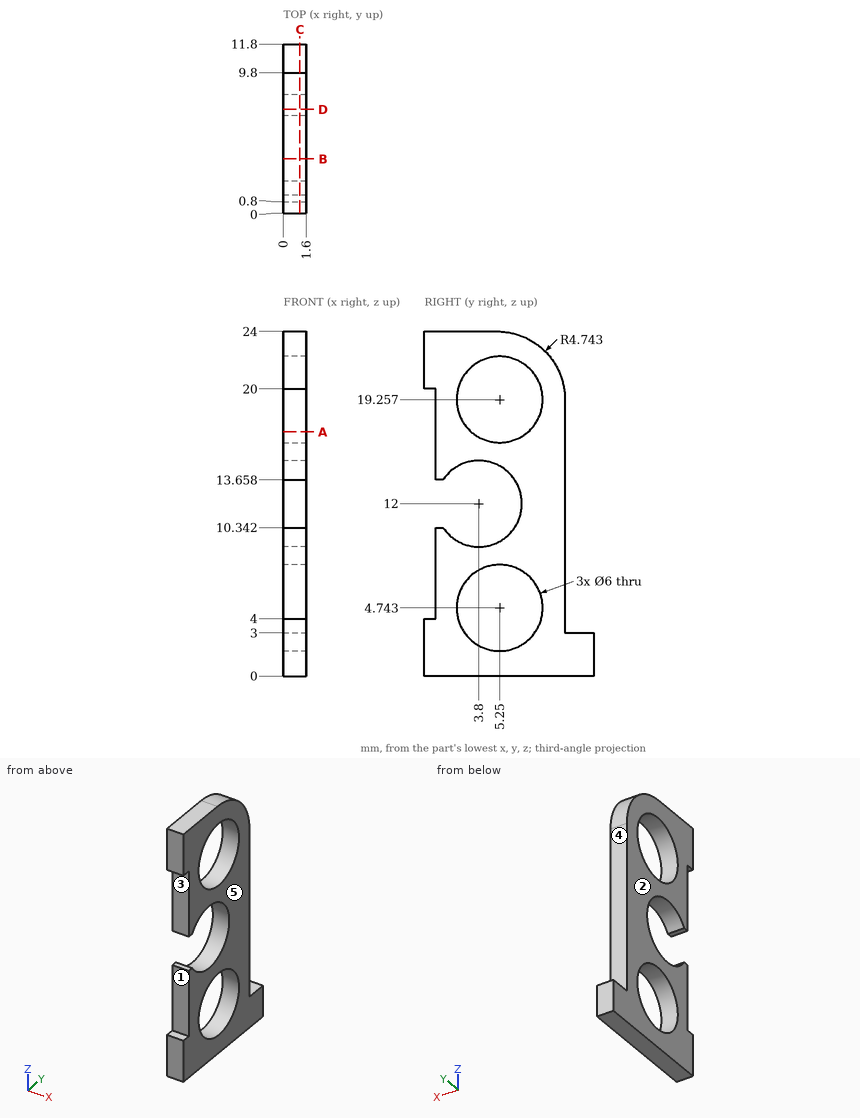
For this review, use the dimensioned drawing (mm, ordinates from the lowest corner) and the shaded views. A direction names the side the tool comes from. Round coordinates to 2 decimals unless told otherwise and drop trailing zeros. Order: outer loops, then holes, each group sorted by start corner. A loop starts at its lowest first (then second) coordinate and runs counter-clockwise, first axis right, second up. Notation, with made-up numbers: M -8.5,75 L 45.5,75 A30 ccw 45.5,110 Z; hole C 64,19.5 d6. An arc over 180 degrees is marked long. Use a Markdown table: item, result. Add a question column.
Item 1: Tool access review of the marked faces 3, 4 and 5: name each direction out of +Z, -Z, +X, -X, +Y, -Y from which nothing blocks a thin tool from reaching the whole face with its end or side.
Item 2: Add section A-A, the plane z = 17. Give the boundary of the cut face in (x, y).
Item 3: To check wall thickness, follow line 1 along Z through (x, y) = (0.55, 1.25); line 2 along Z through (x, y) = (0.55, 4.25) (1 decimal); line 3 along Z through (x, y) = (0.85, 11.25). State the ranges of each line that lie inside material, in increasing order.
Item 4: Add section B-B, the plane y = 3.8. Give the boundary of the cut face in (x, z), then the cut area to 3 significant figures.
Item 5: Add section C-C, the plane x = 1.15. Give the boundary of the cut face in (y, z), then the cut area to 3 significant figures.
Item 6: Insertion check: pin 1 (5 mm diameter, centred on y = 3.8, z = 12, fed in from -X). The pin has a flat end and moves straight along its axis. Give the tip position at first contact, or say it passes through.
Item 7: Add section D-D, the plane y = 7.25. Give the boundary of the cut face in (x, z).
Item 8: Mouldability with a two-part tool opening along Z and no side actions: class the marked faces 1 and 2 as released by +Z, released by -Z, zero draft, split by the parting line, or undercut.
Geometry results:
| question | item | result |
|---|---|---|
| 1 | face 3 | +X, -X, -Y |
| 1 | face 4 | +Z, +X, -X, +Y |
| 1 | face 5 | +Z, -Z, +X, +Y, -Y |
| 2 | outline | M 0,0.8 L 1.6,0.8 L 1.6,3.27 L 0,3.27 Z; M 0,7.23 L 1.6,7.23 L 1.6,9.8 L 0,9.8 Z |
| 3 | line 1 | z = 0 to 10.34, 13.66 to 24 |
| 3 | line 2 | z = 0 to 1.9, 7.6 to 9, 15 to 16.4, 22.1 to 24 |
| 3 | line 3 | z = 0 to 3 |
| 4 | outline | M 0,0 L 1.6,0 L 1.6,2.12 L 0,2.12 Z; M 0,7.37 L 1.6,7.37 L 1.6,9 L 0,9 Z; M 0,15 L 1.6,15 L 1.6,16.63 L 0,16.63 Z; M 0,21.88 L 1.6,21.88 L 1.6,24 L 0,24 Z |
| 4 | area | 12.0 mm² |
| 5 | outline | M 0,0 L 11.8,0 L 11.8,3 L 9.8,3 L 9.8,19.26 A4.74 ccw 5.06,24 L 0,24 L 0,20 L 0.8,20 L 0.8,13.66 L 1.3,13.66 A3 cw long 1.3,10.34 L 0.8,10.34 L 0.8,4 L 0,4 Z; hole C 5.25,4.74 d6; hole C 5.25,19.26 d6 |
| 5 | area | 138 mm² |
| 6 | pin 1 | passes through |
| 7 | outline | M 0,0 L 1.6,0 L 1.6,2.51 L 0,2.51 Z; M 0,6.98 L 1.6,6.98 L 1.6,17.02 L 0,17.02 Z; M 0,21.49 L 1.6,21.49 L 1.6,23.46 L 0,23.46 Z |
| 8 | face 1 | undercut |
| 8 | face 2 | zero draft |
